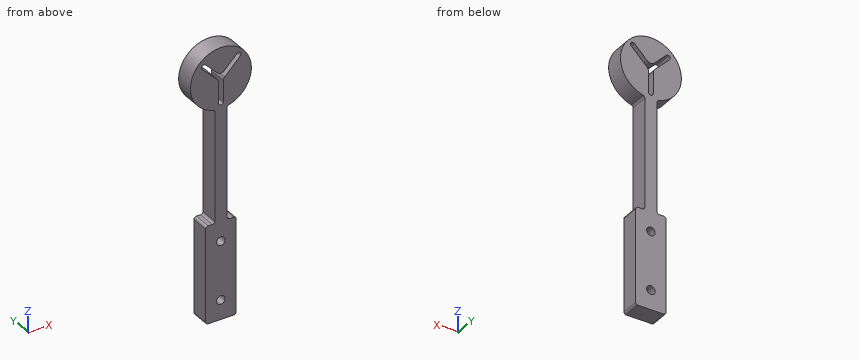
```python
from build123d import *

# Parameters (mm, degrees)
BOSS_EXTRUDE1_DEPTH = 9.525
SKETCH2_R           = 2.2479
CUT_EXTRUDE1_DEPTH  = 10.525
CUT_EXTRUDE2_DEPTH  = 10.525
FILLET1_R           = 1.25
FILLET2_R           = 2.54


with BuildPart() as part:
    # Sketch1 → Boss-Extrude1 (new body)
    with BuildSketch(Plane(origin=(0, 0, 0), x_dir=(1, 0, 0), z_dir=(0, 1, 0))):
        with BuildLine():
            Line((-7.9375, 50.8), (7.9375, 50.8))
            Line((7.9375, 50.8), (7.9375, 0))
            Line((7.9375, 0), (3.175, 0))
            Line((3.175, 0), (3.175, -58.867740133))
            ThreePointArc((3.175, -58.867740133), (0, -90.297), (-3.175, -58.867740133))
            Line((-3.175, -58.867740133), (-3.175, 0))
            Line((-3.175, 0), (-7.9375, 0))
            Line((-7.9375, 0), (-7.9375, 50.8))
        make_face()
    extrude(amount=BOSS_EXTRUDE1_DEPTH)

    # Sketch2 → Cut-Extrude1 (cut, through all)
    with BuildSketch(Plane(origin=(0, 9.525, 0), x_dir=(1, 0, 0), z_dir=(0, 1, 0))):
        with Locations((0, 40.64)):
            Circle(SKETCH2_R)
        with Locations((0, 10.16)):
            Circle(SKETCH2_R)
    extrude(amount=-CUT_EXTRUDE1_DEPTH, mode=Mode.SUBTRACT)

    # Sketch3 → Cut-Extrude2 (cut, through all)
    with BuildSketch(Plane(origin=(0, 9.525, 0), x_dir=(1, 0, 0), z_dir=(0, 1, 0))):
        with BuildLine():
            Line((0.059974982, -75.919115272), (8.472150299, -84.331290589))
            ThreePointArc((8.472150299, -84.331290589), (10.232280498, -84.331290589), (10.232280498, -82.571160389))
            Line((10.232280498, -82.571160389), (1.2446, -73.583479891))
            Line((1.2446, -73.583479891), (1.2446, -61.722))
            ThreePointArc((1.2446, -61.722), (0, -60.4774), (-1.2446, -61.722))
            Line((-1.2446, -61.722), (-1.2446, -73.703429855))
            Line((-1.2446, -73.703429855), (-9.716750299, -82.175580154))
            ThreePointArc((-9.716750299, -82.175580154), (-9.716750299, -83.935710353), (-7.956620099, -83.935710353))
            Line((-7.956620099, -83.935710353), (0.059974982, -75.919115272))
        make_face()
    extrude(amount=-CUT_EXTRUDE2_DEPTH, mode=Mode.SUBTRACT)

    # Fillet1
    fillet1_edges = [part.edges().sort_by_distance(p)[0] for p in [
        (-7.9375, 4.7625, -50.8),
        (7.9375, 4.7625, -50.8),
        (7.9375, 4.7625, 0),
        (3.175, 4.7625, 0),
        (3.175, 4.7625, 58.867740133),
        (-3.175, 4.7625, 58.867740133),
        (-3.175, 4.7625, 0),
        (-7.9375, 4.7625, 0),
    ]]
    fillet(fillet1_edges, radius=FILLET1_R)

    # Fillet2
    fillet2_edges = [part.edges().sort_by_distance(p)[0] for p in [
        (1.2446, 4.7625, 73.583479891),
        (0.059974982, 4.7625, 75.919115272),
        (-1.2446, 4.7625, 73.703429855),
    ]]
    fillet(fillet2_edges, radius=FILLET2_R)


solid = part.part
```
Design review of the part built by this model. Coordinates are the model's own, in mm. Coordinates: 2 decimals unless noted, no trailing zeros. Order: outer loops, then holes, each group sorted by start corner. A loop starts at its lowest first (then second) coordinate and runs counter-clockwise, first axis right, second up.
1) Take a section at A-A, the plane z = -40.64. Give the boundary of the cut face in (x, y) (1 decimal), and give its area (3 significant figures).
2) Clearance check with flat-ended pins moving along their axes: pin 1 (4 mm diameter, centred on x = -7.5, y = 6, fed in from +Z); pin 2 (5 mm diameter, centred on y = 7.5, z = 48.5, fed in from -X) (3 decimals); pin 3 (1.8 mm diameter, centred on x = 6, y = 6.5, fed in from +Z). State where each tip first meets the part, or that it passes through.
3) Take a section at B-B, the plane y = 3.25. State how many separate pieces and enclosed holes the cut face has, and give its area (3 significant figures).
4) Take a section at D-D, the plane z = 66.5. Give the boundary of the cut face in (x, y) (3 decimals), and give its area (3 significant figures).
5) Wall thickness on line 1 along Z through (x, y) = (0, 4.25); line 2 along Z through (x, y) = (-5, 5); line 3 along Z through (x, y) = (4.5, 8.25): over which ranges is each line inside the solid? List them lowest first.
6) Take a section at C-C, the plane x = 0. Give the boundary of the cut face in (y, z) (3 decimals).
Returned:
1. outline: (-7.9, 0) - (-2.2, 0) - (-2.2, 9.5) - (-7.9, 9.5) - close; (2.2, 0) - (7.9, 0) - (7.9, 9.5) - (2.2, 9.5) - close
1. area: 108 mm2
2. pin 1: stops at z = 89.31
2. pin 2: stops at x = -3.175
2. pin 3: stops at z = 89.46
3. separate pieces: 1
3. enclosed holes: 3
3. area: 1,840 mm2
4. outline: (-13.757, 0) - (-1.245, 0) - (-1.245, 9.525) - (-13.757, 9.525) - close; (1.245, 0) - (13.757, 0) - (13.757, 9.525) - (1.245, 9.525) - close
4. area: 238 mm2
5. line 1: z = -50.8 to -42.89, -38.39 to -12.41, -7.91 to 60.48, 76.97 to 90.3
5. line 2: z = -50.8 to 0, 59.35 to 77.46, 80.98 to 89.49
5. line 3: z = -50.8 to 0, 59.2 to 76.84, 80.36 to 89.65
6. outline: (0, -50.8) - (9.525, -50.8) - (9.525, -42.888) - (0, -42.888) - close; (0, -38.392) - (9.525, -38.392) - (9.525, -12.408) - (0, -12.408) - close; (0, -7.912) - (9.525, -7.912) - (9.525, 60.477) - (0, 60.477) - close; (0, 76.972) - (9.525, 76.972) - (9.525, 90.297) - (0, 90.297) - close
